```python
from build123d import *

# Parameters (mm, degrees)
SKETCH2_W                  = 76.2
SKETCH2_H                  = 50.8
BOSS_EXTRUDE2_DEPTH        = 6.35
F_10_32_TAPPED_HOLE1_D     = 4.0386
F_10_32_TAPPED_HOLE1_DEPTH = 12.02944
F_10_32_TAPPED_HOLE1_TIP   = 1.213317848
SKETCH6_R                  = 14.2875
CUT_EXTRUDE1_DEPTH         = 47.228697797
F_10_CLEARANCE_HOLE1_D     = 5.1054
SKETCH13_W                 = 10.345899722
SKETCH13_H                 = 50.8
CUT_EXTRUDE2_DEPTH         = 47.228697797
FILLET3_R                  = 25.4


with BuildPart() as part:
    # Sketch2 → Boss-Extrude2 (new body)
    with BuildSketch(Plane(origin=(0, 0, 0), x_dir=(0, 0, -1), z_dir=(1, 0, 0))):
        Rectangle(SKETCH2_W, SKETCH2_H)
    extrude(amount=BOSS_EXTRUDE2_DEPTH)

    # #10-32 Tapped Hole1
    with Locations(Plane.XY.offset(38.1)):
        with Locations((3.175, -12.7), (3.175, 0), (3.175, 12.7)):
            Hole(F_10_32_TAPPED_HOLE1_D / 2, depth=F_10_32_TAPPED_HOLE1_DEPTH)
            with Locations((0, 0, -(F_10_32_TAPPED_HOLE1_DEPTH + F_10_32_TAPPED_HOLE1_TIP / 2))):  # 118° drill point
                Cone(0, F_10_32_TAPPED_HOLE1_D / 2, F_10_32_TAPPED_HOLE1_TIP, mode=Mode.SUBTRACT)

    # Sketch6 → Cut-Extrude1 (cut, through all)
    with BuildSketch(Plane(origin=(6.35, 0, 0), x_dir=(0, 0, -1), z_dir=(1, 0, 0))):
        with Locations((-6.35, 0)):
            Circle(SKETCH6_R)
    extrude(amount=-CUT_EXTRUDE1_DEPTH, mode=Mode.SUBTRACT)

    # #10 Clearance Hole1 (through all)
    with Locations(Plane.ZY):
        with Locations((-8.704100278, -20.440822776), (21.413163559, 20.468716687), (21.413163559, -20.468716687), (-8.704100278, 20.440822776)):
            Hole(F_10_CLEARANCE_HOLE1_D / 2)

    # Sketch13 → Cut-Extrude2 (cut, through all)
    with BuildSketch(Plane(origin=(6.35, 0, 0), x_dir=(0, 0, -1), z_dir=(1, 0, 0))):
        with Locations((32.927050139, 0)):
            Rectangle(SKETCH13_W, SKETCH13_H)
    extrude(amount=-CUT_EXTRUDE2_DEPTH, mode=Mode.SUBTRACT)

    # Fillet3
    fillet3_edges = [part.edges().sort_by_distance(p)[0] for p in [
        (3.175, 25.4, -27.754100278),
        (3.175, -25.4, -27.754100278),
    ]]
    fillet(fillet3_edges, radius=FILLET3_R - 0.0001)  # a hair under: the kernel refuses the full size


solid = part.part
```
Model file for the job. Use its own axes, mm. A direction names the side the tool comes from. Coordinates: 2 decimals unless noted, no trailing zeros. Order: outer loops, then holes, each group sorted by start corner. A loop starts at its lowest first (then second) coordinate and runs counter-clockwise, first axis right, second up. Notation, with made-up numbers: (14.25, 62) -> (24.25, 62) arc R16 cw to (24.25, 82) -> close; hole circle Ø2 at (81.5, 18.25). An arc over 180 degrees is marked (long way). Answer as a JSON object with one key per item and string values. Group by question number.
1) Cut at B-B, the plane z = 34. Write the cut outline in (x, y) (3 decimals), then the cut area to 3 significant figures.
2) Drill centre lines: L1, parallel to Y at x = 3, z = 35; L2, parallel to X at y = -12.7, z = 34.5; L3, parallel to Y at x = 1.75, z = 19.5. Where is each one in solid material? Low to high.
3) Cut at D-D, the plane z = -9. Write the cut outline in (x, y), then the cut area to 3 significant figures.
4) Flat gauge pins, fed straight in: pin 1 (17 mm diameter, centred on y = 0, z = 6.35, fed in from +X); pin 2 (3.5 mm diameter, centred on x = 3.175, y = 12.7, fed in from -Z); pin 3 (3 mm diameter, centred on x = 3.175, y = -12.7, fed in from +Z); pin 4 (1.5 mm diameter, centred on x = 5.5, z = -15.5, fed in from -Y). Where does each tip first touch, or does it go through?
5) Cut at C-C, the plane y = 8.5. Write the cut outline in (x, z).
6) Which spindle directions (+Z, -Z, +X, -X, +Y, -Y) get a long thin tool onto all of the face, cutting with end or side? Do faces 4 (the face through (3.22, -17.91, -8.37)), 5 (the face through (4.8, 11.5, 32)). Say none if no direction does.
7) Cut at A-A, the plane z = 6.35. Write the cut outline in (x, y).
8) Pull direction X, two halves, no side cores. Call faces 1 (the face through (6.35, 6, 20)), 2 (the face through (1.25, 0.61, 32)), 3 (the face through (3.22, 22.62, 20.04)): +X half, -X half, draft (parallel to the pull), parting line (faces both ways), or undercut.
Check values:
{
 "1": {"outline": "(0, -25.4) -> (6.35, -25.4) -> (6.35, 25.4) -> (0, 25.4) -> close; hole circle Ø4.039 at (3.175, -12.7); hole circle Ø4.039 at (3.175, 0); hole circle Ø4.039 at (3.175, 12.7)", "area": "284 mm²"},
 "2": {"L1": "y = -25.4 to -14.71, -10.69 to -2.01, 2.01 to 10.69, 14.71 to 25.4", "L2": "x = 0 to 1.16, 5.19 to 6.35", "L3": "y = -25.4 to -22.16, -18.78 to -5.59, 5.59 to 18.78, 22.16 to 25.4"},
 "3": {"outline": "(0, -24.52) -> (6.35, -24.52) -> (6.35, -22.98) -> (0, -22.98) -> close; (0, -17.91) -> (6.35, -17.91) -> (6.35, 17.91) -> (0, 17.91) -> close; (0, 22.98) -> (6.35, 22.98) -> (6.35, 24.52) -> (0, 24.52) -> close", "area": "247 mm²"},
 "4": {"pin 1": "passes through", "pin 2": "stops at z = -25.27", "pin 3": "stops at z = 25.76", "pin 4": "stops at y = -22.17"},
 "5": {"outline": "(0, -26.29) -> (6.35, -26.29) -> (6.35, -5.13) -> (0, -5.13) -> close; (0, 17.83) -> (6.35, 17.83) -> (6.35, 38.1) -> (0, 38.1) -> close"},
 "6": {"face 4": "+X, -X", "face 5": "+Z"},
 "7": {"outline": "(0, -25.4) -> (6.35, -25.4) -> (6.35, -14.29) -> (0, -14.29) -> close; (0, 14.29) -> (6.35, 14.29) -> (6.35, 25.4) -> (0, 25.4) -> close"},
 "8": {"face 1": "+X half", "face 2": "undercut", "face 3": "draft"}
}
